Input: dimensioned drawing with shaded views. Units: mm. Origin: part minimum x, y, z. Coordinates: 2 decimals unless noted, no trailing zeros. Loops run counter-clockwise (first coordinate to the right, second up) from the corner with the lowest first, then second, coordinate; pieces in that order, holes last.
Item 1: Section C-C on z = 17. Return loops of the section in (x, y), and give its area (3 significant figures).
Item 2: Section B-B on y = 1.05. Return loops of the section in (x, z), and give its area (3 significant figures).
Item 3: Pull-direction query (X, two-part tool) for the marked faces 1, 2, 3 and 4; classes: released by +X, released by -X, zero draft, split by the parting line, or undercut.
Item 4: Section A-A on x = 4. Return loops of the section in (y, z).
Item 5: Ray query, line 1 along Z through (x, y) = (4, 1.9); line 2 along X through (y, z) = (0.9, 3); line 3 along X through (y, z) = (0.3, 2). Return the intervals inside material, ascending.
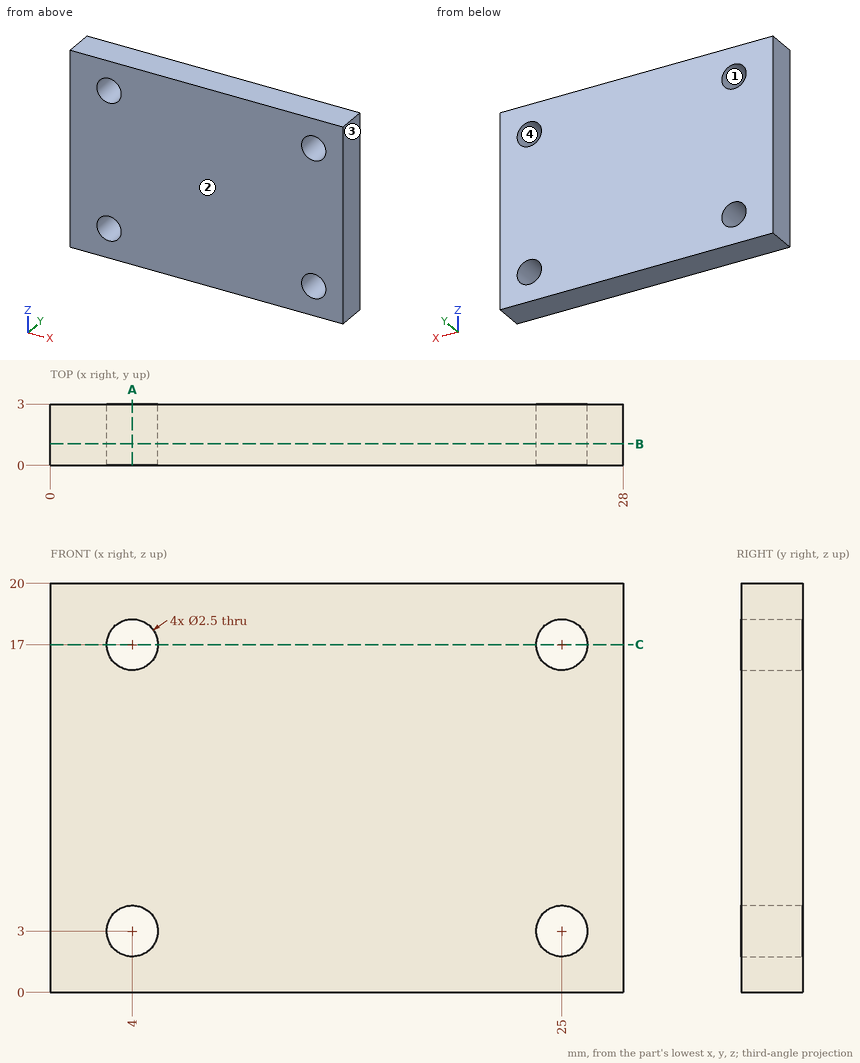
Results found:
1. outline: (0, 0) - (2.75, 0) - (2.75, 3) - (0, 3) - close; (5.25, 0) - (23.75, 0) - (23.75, 3) - (5.25, 3) - close; (26.25, 0) - (28, 0) - (28, 3) - (26.25, 3) - close
1. area: 69.0 mm2
2. outline: (0, 0) - (28, 0) - (28, 20) - (0, 20) - close; hole circle Ø2.5 at (4, 3); hole circle Ø2.5 at (4, 17); hole circle Ø2.5 at (25, 3); hole circle Ø2.5 at (25, 17)
2. area: 540 mm2
3. face 1: undercut
3. face 2: zero draft
3. face 3: released by +X
3. face 4: undercut
4. outline: (0, 0) - (3, 0) - (3, 1.75) - (0, 1.75) - close; (0, 4.25) - (3, 4.25) - (3, 15.75) - (0, 15.75) - close; (0, 18.25) - (3, 18.25) - (3, 20) - (0, 20) - close
5. line 1: z = 0 to 1.75, 4.25 to 15.75, 18.25 to 20
5. line 2: x = 0 to 2.75, 5.25 to 23.75, 26.25 to 28
5. line 3: x = 0 to 3.25, 4.75 to 24.25, 25.75 to 28
